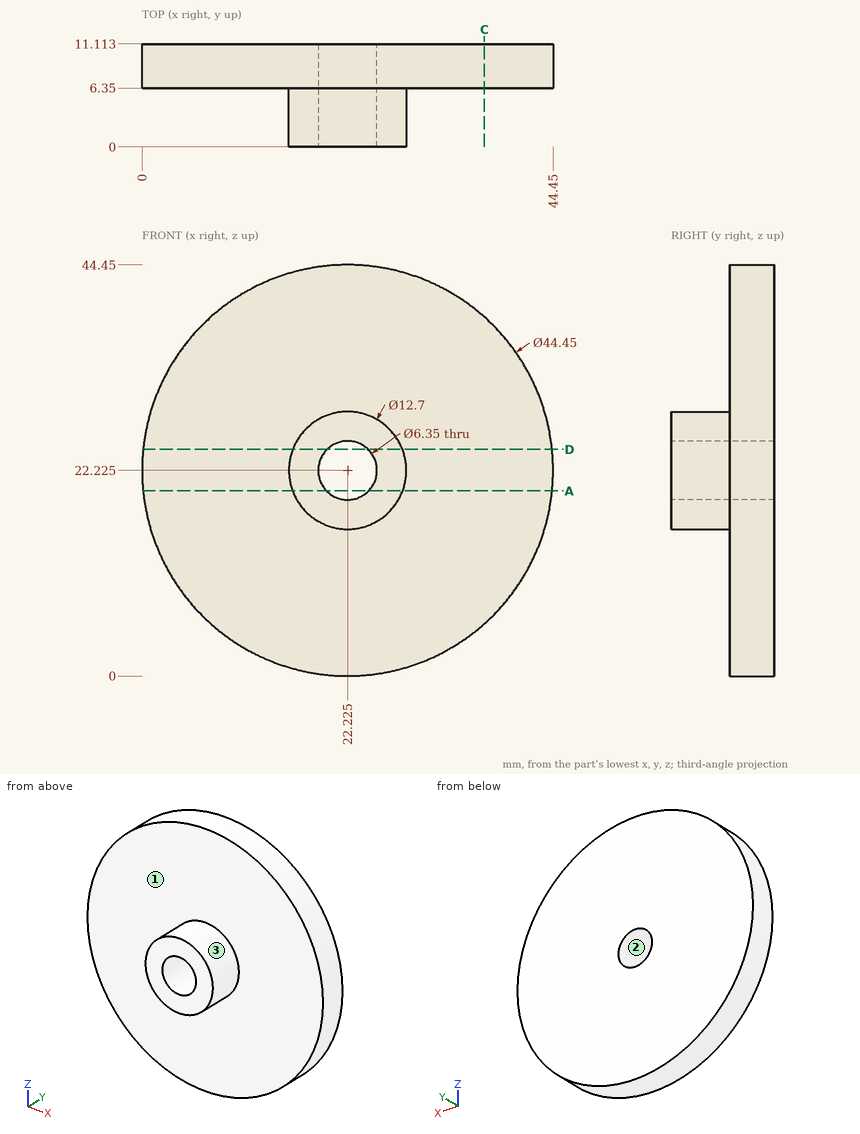
The figure shows three views and two pictorial views of one solid part (mm, origin at its lowest corner). Answer the questions. Coordinates: 2 decimals unless noted, no trailing zeros. Loops run counter-clockwise (first coordinate to the right, second up) from the corner with the lowest first, then second, coordinate; pieces in that order, holes last. Notation, with made-up numbers: (72.25, 49) -> (78.25, 49) arc R11 cw to (78.25, 56) -> close; hole circle Ø10 at (80, 26). An arc over 180 degrees is marked (long way). Return JSON: item names as keys, results as strings. Group by question number.
(1) A cutting plane is placed at D-D on z = 24.5. Write down the section's boundary in (x, y).
(2) Determine the mould class of the marked faces 1, 2 and 3 for opening direction Z: released by +Z, released by -Z, zero draft, split by the parting line, or undercut.
(3) A cutting plane is placed at A-A on z = 20. Write down the section's boundary in (x, y).
(4) Given pin 1 Ø2 at (x, z) = (24.5, 36.5) entering from -Y; pin 2 Ø5 at (y, z) = (7.5, 11.5) entering from -X; pin 3 Ø6 at (y, z) = (3, 38.5) entering from +X, each flat-ended and moving along its own axis, determine where each tip first touches the part or whether it passes through.
(5) A cutting plane is placed at C-C on x = 37. Write down the section's boundary in (y, z), and give its area (3 significant figures).
(6) Find the intervals of material crossed by probe 1 along Y at (x, z) = (37.5, 8.5); probe 2 along X at (y, z) = (9, 22); probe 3 along Z at (x, y) = (25, 7.25) (1 decimal), in increasing order. Write a range as from..to.
The answers:
{
 "1": {"outline": "(0.12, 6.35) -> (16.3, 6.35) -> (16.3, 0) -> (20.01, 0) -> (20.01, 11.11) -> (0.12, 11.11) -> close; (24.44, 0) -> (28.15, 0) -> (28.15, 6.35) -> (44.33, 6.35) -> (44.33, 11.11) -> (24.44, 11.11) -> close"},
 "2": {"face 1": "zero draft", "face 2": "undercut", "face 3": "split by the parting line"},
 "3": {"outline": "(0.11, 6.35) -> (16.28, 6.35) -> (16.28, 0) -> (19.96, 0) -> (19.96, 11.11) -> (0.11, 11.11) -> close; (24.49, 0) -> (28.17, 0) -> (28.17, 6.35) -> (44.34, 6.35) -> (44.34, 11.11) -> (24.49, 11.11) -> close"},
 "4": {"pin 1": "stops at y = 6.35", "pin 2": "stops at x = 1.58", "pin 3": "passes through"},
 "5": {"outline": "(6.35, 5.62) -> (11.11, 5.62) -> (11.11, 38.83) -> (6.35, 38.83) -> close", "area": "158 mm^2"},
 "6": {"probe 1": "y = 6.35..11.11", "probe 2": "x = 0..19.06, 25.39..44.45", "probe 3": "z = 0.2..20.7, 23.8..44.3"}
}
